from build123d import *

# Parameters (mm, degrees)
SKETCH1_R                     = 3
BOSS_EXTRUDE1_DEPTH           = 4
SKETCH2_W                     = 0.65
SKETCH2_H                     = 0.65
CUT_EXTRUDE1_DEPTH            = 2.5
CIRPATTERN1_COUNT             = 25
SKETCH3_OUTSIDE_W             = 9.876
SKETCH3_OUTSIDE_H             = 9.876
SKETCH3_OUTSIDE_R             = 2.5
CUT_EXTRUDE2_DEPTH            = 0.5
CSK_FOR_M3_SFHCS1_D           = 1.5
CSK_FOR_M3_SFHCS1_CSINK_D     = 2
CSK_FOR_M3_SFHCS1_CSINK_ANGLE = 90


with BuildPart() as part:
    # Sketch1 → Boss-Extrude1 (new body)
    with BuildSketch(Plane(origin=(0, 0, 0), x_dir=(1, 0, 0), z_dir=(0, 1, 0))):
        Circle(SKETCH1_R)
    extrude(amount=BOSS_EXTRUDE1_DEPTH)

    # Sketch2 → Cut-Extrude1 (cut)
    with BuildSketch(Plane(origin=(0, 4, 0), x_dir=(1, 0, 0), z_dir=(0, 1, 0))):
        with Locations((2.121320344, 2.121320344)):
            Rectangle(SKETCH2_W, SKETCH2_H)
    cut_extrude1 = extrude(amount=-CUT_EXTRUDE1_DEPTH, mode=Mode.SUBTRACT)

    # CirPattern1: Cut-Extrude1 ×25 about axis
    cirpattern1_axis = Axis((0, 0, 0), (0, 1, 0))
    for i in range(1, CIRPATTERN1_COUNT):
        add(cut_extrude1.rotate(cirpattern1_axis, i * 360 / CIRPATTERN1_COUNT), mode=Mode.SUBTRACT)

    # Sketch3 outside → Cut-Extrude2 (cut)
    with BuildSketch(Plane(origin=(0, 1.5, 0), x_dir=(1, 0, 0), z_dir=(0, 1, 0))):
        Rectangle(SKETCH3_OUTSIDE_W, SKETCH3_OUTSIDE_H)
        Circle(SKETCH3_OUTSIDE_R, mode=Mode.SUBTRACT)
    extrude(amount=-CUT_EXTRUDE2_DEPTH, mode=Mode.SUBTRACT)

    # CSK for M3 SFHCS1 (through all)
    with Locations(Plane(origin=(0, 4, 0), x_dir=(1, 0, 0), z_dir=(0, 1, 0))):
        with Locations((0, 0)):
            CounterSinkHole(CSK_FOR_M3_SFHCS1_D / 2, CSK_FOR_M3_SFHCS1_CSINK_D / 2, counter_sink_angle=CSK_FOR_M3_SFHCS1_CSINK_ANGLE)


solid = part.part
Build history of the part. All positions in model axes, mm. A direction names the side the tool comes from. Coordinates: 2 decimals unless noted, no trailing zeros. Order: outer loops, then holes, each group sorted by start corner. A loop starts at its lowest first (then second) coordinate and runs counter-clockwise, first axis right, second up. Notation, with made-up numbers: M 22.5,35 L 53.5,35 A9 ccw 53.5,51 Z; hole C -31,88 d9. An arc over 180 degrees is marked long. One line per question, with ' | ' between items. Start each with the question number.
Q1. Two-plate mould, pull along X, no slides. Class faces 1 (the face through (-3, 0.5, -0.1)), 2 (the face through (0.75, 1.85, -0.03)), 3 (the face through (-2, 1, -2)): +X half, -X half, draft (parallel to the pull), parting line (faces both ways), or undercut.
Q2. 3-axis set-ups, long thin cutter, end or side, ignore diameter. For faces 4 (the face through (0, 4, 1.3)), 5 (the face through (-0.54, 1.25, 2.44)): which of +Z, -Z, +X, -X, +Y, -Y reach the whole face in a straight line?
Q3. Saw through at A-A (x = 0). List the corners of the cut face in (y, z).
Q4. Saw through at C-C (z = 0). List the corners of the cut face in (x, y), then the cut area to 3 significant figures.
Q5. Flat gauge pins, fed straight in: pin 1 Ø0.6 at (x, y) = (2, 2) entering from -Z; pin 2 Ø3 at (x, z) = (-1.5, 0) entering from -Y; pin 3 Ø1.5 at (x, y) = (-2.5, 1) entering from +Z; pin 4 Ø1.5 at (x, y) = (1, 1.5) entering from +Z. Where does each tip first touch, or does it go through?
Q6. Probe L1, parallel to Y at x = 0.45, z = 2.55; L2, parallel to Z at x = 0.3, y = 1.8; L3, parallel to X at y = 1.35, z = -0.15. List the from-to ranges inside material, lowest first. Write a range as from..to.
Q7. Saw through at B-B (y = 0.45). List the corners of the cut face in (x, z), then the cut area to 3 significant figures.
Check values:
1) face 1: parting line | face 2: undercut | face 3: draft
2) face 4: +Z, -Z, +X, -X, +Y | face 5: none
3) outline: M 0,-3 L 1,-3 L 1,-2.5 L 1.5,-2.5 L 1.5,-2.62 L 4,-2.62 L 4,-1 L 3.75,-0.75 L 0,-0.75 Z; M 0,0.75 L 3.75,0.75 L 4,1 L 4,2.82 L 1.5,2.82 L 1.5,2.5 L 1,2.5 L 1,3 L 0,3 Z
4) outline: M -3,0 L -0.75,0 L -0.75,3.75 L -1,4 L -2.82,4 L -2.82,1.5 L -2.5,1.5 L -2.5,1 L -3,1 Z; M 0.75,0 L 3,0 L 3,1 L 2.5,1 L 2.5,1.5 L 2.62,1.5 L 2.62,4 L 1,4 L 0.75,3.75 Z | area: 16.0 mm2
5) pin 1: stops at z = -2.32 | pin 2: stops at y = 0 | pin 3: stops at z = 2.44 | pin 4: stops at z = 2.97
6) L1: y = 0..1, 1.5..4 | L2: z = -2.75..-0.69, 0.69..2.58 | L3: x = -2.5..-0.73, 0.73..2.5
7) outline: C 0,0 d6; hole C 0,0 d1.5 | area: 26.5 mm2
